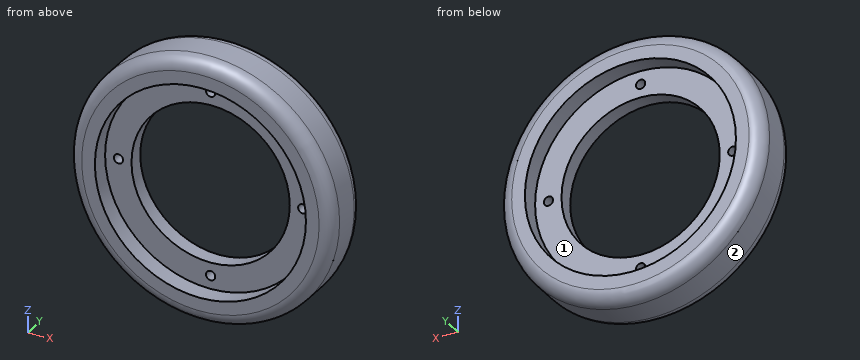
from build123d import *

# Parameters (mm, degrees)
F0_R      = 63.5
F1_DEPTH  = 12.7
F2_R      = 6.35
F3_R      = 50.8
F4_DEPTH  = 8.89
F5_R      = 50.8
F6_DEPTH  = 8.89
F7_R      = 38.1
F8_DEPTH  = 25.401
F9_R      = 2.230901
F10_DEPTH = 16.511


with BuildPart() as f1:
    # F0 (on Front) → F1 (new body, symmetric)
    with BuildSketch(Plane.XZ):
        Circle(F0_R)
    extrude(amount=F1_DEPTH, both=True)

    # F2
    f2_edges = [f1.edges().sort_by_distance(p)[0] for p in [
        (-63.5, -12.7, 0),
        (-63.5, 12.7, 0),
    ]]
    fillet(f2_edges, radius=F2_R)

    # F3 (on face) → F4 (cut)
    with BuildSketch(Plane.XZ.offset(12.7)):
        Circle(F3_R)
    extrude(amount=-F4_DEPTH, mode=Mode.SUBTRACT)

    # F5 (on face) → F6 (cut)
    with BuildSketch(Plane(origin=(0, 12.7, 0), x_dir=(-1, 0, 0), z_dir=(0, 1, 0))):
        Circle(F5_R)
    extrude(amount=-F6_DEPTH, mode=Mode.SUBTRACT)

    # F7 (on face) → F8 (cut, through all)
    with BuildSketch(Plane.XZ.offset(12.7)):
        Circle(F7_R)
    extrude(amount=-F8_DEPTH, mode=Mode.SUBTRACT)

    # F9 (on face) → F10 (cut, through all)
    with BuildSketch(Plane.XZ.offset(3.81)):
        with Locations((-44.369552, 0)):
            Circle(F9_R)
        with Locations((0, 44.369552)):
            Circle(F9_R)
        with Locations((44.369552, 0)):
            Circle(F9_R)
        with Locations((0, -44.369552)):
            Circle(F9_R)
    extrude(amount=-F10_DEPTH, mode=Mode.SUBTRACT)


solid = f1.part
Check sheet for the modelled part. Datum: model origin and axes. Units: mm. Face numbers are marked on the shaded views. Round coordinates to 2 decimals unless told otherwise and drop trailing zeros. Order: outer loops, then holes, each group sorted by start corner. A loop starts at its lowest first (then second) coordinate and runs counter-clockwise, first axis right, second up.
Q1. Depth check by flat-ended pin: P1, Ø3, axis at y = 1.5, z = -15, coming from the -X side; P2, Ø2, axis at x = 17.5, y = 5.5, coming from the +Z side; P3, Ø8, axis at y = 9, z = -25.5, coming from the -X side. Enter the tip coordinate at first touch or a pass-through.
Filled sheet:
P1: stops at x = -62.05
P2: stops at z = 61.32
P3: stops at x = -59.54
Q2. Cross-section at B-B, the plane z = 0. Enter the section's corners in (x, y), plus the area to 3 significant figures.
Filled sheet:
outline: (-63.5, -6.35) arc R6.35 ccw to (-57.15, -12.7) - (-50.8, -12.7) - (-50.8, -3.81) - (-46.6, -3.81) - (-46.6, 3.81) - (-50.8, 3.81) - (-50.8, 12.7) - (-57.15, 12.7) arc R6.35 ccw to (-63.5, 6.35) - close; (-42.14, -3.81) - (-38.1, -3.81) - (-38.1, 3.81) - (-42.14, 3.81) - close; (38.1, -3.81) - (42.14, -3.81) - (42.14, 3.81) - (38.1, 3.81) - close; (46.6, -3.81) - (50.8, -3.81) - (50.8, -12.7) - (57.15, -12.7) arc R6.35 ccw to (63.5, -6.35) - (63.5, 6.35) arc R6.35 ccw to (57.15, 12.7) - (50.8, 12.7) - (50.8, 3.81) - (46.6, 3.81) - close
area: 736 mm2
Q3. Scan lines: L1, parallel to Z at x = 0, y = -0.25; L2, parallel to Y at x = 44, z = -4; L3, parallel to X at y = 0.75, z = -3. Record each from-to range of solid material in increasing order.
Filled sheet:
L1: z = -63.5 to -46.6, -42.14 to -38.1, 38.1 to 42.14, 46.6 to 63.5
L2: y = -3.81 to 3.81
L3: x = -63.43 to -37.98, 37.98 to 63.43
Q4. Draft check along Z on the marked faces 1 and 2. Enter one of: pulls with the +Z half, pulls with the -Z half, needs draft (parallel to the pull), parting line crosses it, or undercut.
Filled sheet:
face 1: undercut
face 2: parting line crosses it
Q5. Cross-section at A-A, the plane x = 0. Enter the section's corners in (y, z).
Filled sheet:
outline: (-12.7, -57.15) arc R6.35 ccw to (-6.35, -63.5) - (6.35, -63.5) arc R6.35 ccw to (12.7, -57.15) - (12.7, -50.8) - (3.81, -50.8) - (3.81, -46.6) - (-3.81, -46.6) - (-3.81, -50.8) - (-12.7, -50.8) - close; (-12.7, 50.8) - (-3.81, 50.8) - (-3.81, 46.6) - (3.81, 46.6) - (3.81, 50.8) - (12.7, 50.8) - (12.7, 57.15) arc R6.35 ccw to (6.35, 63.5) - (-6.35, 63.5) arc R6.35 ccw to (-12.7, 57.15) - close; (-3.81, -42.14) - (3.81, -42.14) - (3.81, -38.1) - (-3.81, -38.1) - close; (-3.81, 38.1) - (3.81, 38.1) - (3.81, 42.14) - (-3.81, 42.14) - close
